Verification items for the finished model (mm, model axes). Face numbers are marked on the shaded views. A direction names the side the tool comes from. Coordinates: 2 decimals unless noted, no trailing zeros. Write each loop counter-clockwise with the first axis right and the second up, starting at its lowest first coordinate (ties: lowest second). Pieces come first, ordered by that corner, then holes. Notation, with made-up numbers: M 46.5,15 L 70.5,15 A32 cw 70.5,48 Z; hole C -24,-14.75 d10. An arc over 180 degrees is marked long. One line per item, written item: value.
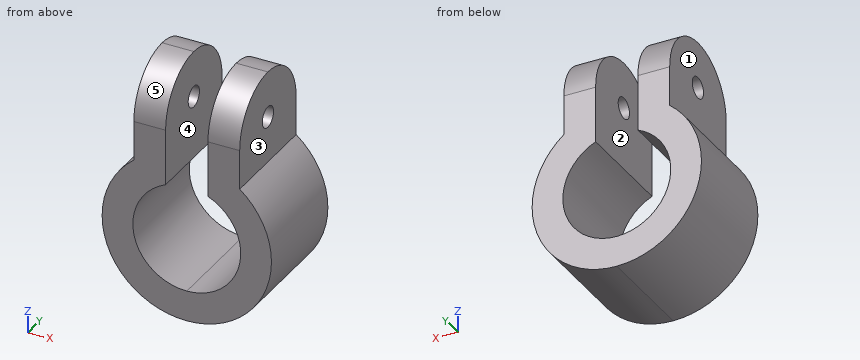
```python
from build123d import *

# Parameters (mm, degrees)
F1_DEPTH = 5
F2_R     = 1
F3_DEPTH = 25
F4_R     = 4.99999


# Not quite as in the source:
# - a fillet or chamfer is up to 0.001 mm smaller than in the source, because OpenCascade refuses the exact size
# - a feature names something its author has since deleted; it is built from what else it names


with BuildPart() as f1:
    # F0 (on Front) → F1 (new body, symmetric)
    with BuildSketch(Plane.XZ):
        with BuildLine():
            ThreePointArc((2, 4.6914816423), (4.9968268119, -1.0206477415), (0, -5.1))
            Line((0, -5.1), (0, -8))
            ThreePointArc((0, -8), (7.5485092564, -2.6495297708), (5, 6.2449979984))
            ThreePointArc((5, 6.2449979984), (3.5795567819, 7.1544932207), (2, 7.7459666924))
            Line((2, 7.7459666924), (2, 4.6914816423))
        make_face()
        with BuildLine():
            Line((2, 15), (2, 7.7459666924))
            ThreePointArc((2, 7.7459666924), (3.5795567819, 7.1544932207), (5, 6.2449979984))
            Line((5, 6.2449979984), (5, 15))
            Line((5, 15), (2, 15))
        make_face()
    extrude(amount=F1_DEPTH, both=True)

    # F2 (on face) → F3 (cut)
    with BuildSketch(Plane.YZ.offset(5)):
        with Locations((0, 10.6224989992)):
            Circle(F2_R)
    extrude(amount=-F3_DEPTH, mode=Mode.SUBTRACT)

    # F4 (radius 5 in the source; OpenCascade refuses exactly that, so slightly less here)
    f4_edges = [f1.edges().sort_by_distance(p)[0] for p in [
        (3.5, -5, 15),
        (3.5, 5, 15),
    ]]
    fillet(f4_edges, radius=F4_R)

    # F5: F1 across plane


with BuildPart() as f1_1:
    add(f1.part)
    add(f1.part.mirror(Plane.YZ))


solid = f1_1.part
```
Item 1: Scan lines: line 1 (Z direction, x = -2.55, y = 0); line 2 (X direction, y = -1, z = 10); line 3 (Z direction, x = -3.85, y = 0). Record each from-to range of solid material in increasing order.
The answers:
line 1: z = -7.58 to -4.42, 4.42 to 9.62, 11.62 to 15
line 2: x = -5 to -2, 2 to 5
line 3: z = -7.01 to -3.34, 3.34 to 9.62, 11.62 to 15
Item 2: Cross-section at C-C, the plane z = -3.5. Enter the section's corners in (x, y).
The answers:
outline: M -7.19,-5 L -3.71,-5 L -3.71,5 L -7.19,5 Z; M 3.71,-5 L 7.19,-5 L 7.19,5 L 3.71,5 Z
Item 3: Draft check along X on the marked faces 1, 2 and 3. Enter one of: released by +X, released by -X, zero draft, split by the parting line, or undercut.
The answers:
face 1: released by -X
face 2: undercut
face 3: released by +X
Item 4: Cross-section at A-A, the plane x = 3.75. Give the number of separate pieces and of enclosed holes in the cut face, and give its area (3 significant figures).
The answers:
separate pieces: 2
enclosed holes: 1
area: 138 mm²
Item 5: Access from +Z, -Z, +X, -X, +Y, -Y to the whole of each face (thin tool, end or side, straight path). Record for the marked faces 4 and 5.
The answers:
face 4: +Z, +Y, -Y
face 5: +Z, +X, -X, -Y
Item 6: Go/stop test with flat-tipped pins: P1, Ø2.5, axis at y = 0, z = 10.62, coming from the +X side; P2, Ø4.5, axis at y = -0.5, z = 10, coming from the -X side; P3, Ø1.5, axis at x = 3, y = -1.5, coming from the -Z side. Record where each tip stops, or that it passes through.
The answers:
P1: stops at x = 5
P2: stops at x = -5
P3: stops at z = -7.68
Item 7: Cross-section at B-B, the plane y = -0.75. Enter the section's corners in (x, z) (3 decimals).
The answers:
outline: M -5,6.245 A8 ccw long 5,6.245 L 5,9.961 L 2,9.961 L 2,4.691 A5.1 cw long -2,4.691 L -2,9.961 L -5,9.961 Z; M -5,11.284 L -2,11.284 L -2,14.943 L -5,14.943 Z; M 2,11.284 L 5,11.284 L 5,14.943 L 2,14.943 Z
